from build123d import *

# Parameters (mm, degrees)
ESQUISSE1_R                                = 30
BOSS_EXTRU_1_DEPTH                         = 15
ESQUISSE2_R                                = 12.5
BOSS_EXTRU_2_DEPTH                         = 69
ESQUISSE4_2_W                              = 230
ESQUISSE4_2_H                              = 40
ENL_V_MAT_EXTRU_1_DEPTH                    = 5
CHAMBRAGE_POUR_VIS_T_TE_HEXAGONALE_2_COUNT = 2
CHAMBRAGE_POUR_VIS_T_TE_HEXAGONALE_2_PITCH = 41
ESQUISSE17_R                               = 6
BOSS_EXTRU_4_DEPTH                         = 88.38
ESQUISSE18_W                               = 10.356322474
ESQUISSE18_H                               = 3
ENL_V_MAT_EXTRU_2_DEPTH                    = 3


with BuildPart() as part:
    # Esquisse1 → Boss.-Extru.1 (new body)
    with BuildSketch(Plane.XY):
        Circle(ESQUISSE1_R)
    extrude(amount=BOSS_EXTRU_1_DEPTH)

    # Esquisse2 → Boss.-Extru.2 (add)
    with BuildSketch(Plane(origin=(0, 0, 0), x_dir=(-1, 0, 0), z_dir=(0, 0, -1))):
        with Locations(Location((0, 0, 0), (0, 0, 180))):
            Circle(ESQUISSE2_R)
    extrude(amount=BOSS_EXTRU_2_DEPTH)

    # Esquisse4<2> → Enlèv. mat.-Extru.1 (cut)
    with BuildSketch(Plane.XY.offset(15)):
        Rectangle(ESQUISSE4_2_W, ESQUISSE4_2_H)
    extrude(amount=-ENL_V_MAT_EXTRU_1_DEPTH, mode=Mode.SUBTRACT)

    # Esquisse14 → Chambrage pour vis à tête hexagonale M51 (revolve, cut)
    with BuildSketch(Plane.YZ.offset(-20.5)):
        Polygon((0, 0), (0, 15), (2.75, 15), (2.75, 3.605), (2.775, 3.58), (6.12, 3.58), (6.12, 0), align=None)
    chambrage_pour_vis_t_te_hexagonale_m51 = revolve(axis=Axis((-20.5, 0, -6.35), (0, 0, 1)), mode=Mode.SUBTRACT)

    # Chambrage pour vis _ t_te hexagonale 2: Chambrage pour vis à tête hexagonale M51 ×2
    with Locations(*[(i * CHAMBRAGE_POUR_VIS_T_TE_HEXAGONALE_2_PITCH, 0, 0) for i in range(1, CHAMBRAGE_POUR_VIS_T_TE_HEXAGONALE_2_COUNT)]):
        add(chambrage_pour_vis_t_te_hexagonale_m51, mode=Mode.SUBTRACT)

    # Esquisse17 → Boss.-Extru.4 (add)
    with BuildSketch(Plane(origin=(0, 0, -69), x_dir=(-1, 0, 0), z_dir=(0, 0, -1))):
        Circle(ESQUISSE17_R)
    extrude(amount=BOSS_EXTRU_4_DEPTH)

    # Esquisse18 → Enlèv. mat.-Extru.2 (cut)
    with BuildSketch(Plane(origin=(0, 0, -157.38), x_dir=(-1, 0, 0), z_dir=(0, 0, -1))):
        with Locations((1.787207702, 0)):
            Rectangle(ESQUISSE18_W, ESQUISSE18_H)
    extrude(amount=-ENL_V_MAT_EXTRU_2_DEPTH, mode=Mode.SUBTRACT)


solid = part.part
Design review of the part built by this model. Coordinates are the model's own, in mm. A direction names the side the tool comes from. Coordinates: 2 decimals unless noted, no trailing zeros. Loops run counter-clockwise (first coordinate to the right, second up) from the corner with the lowest first, then second, coordinate; pieces in that order, holes last. Notation, with made-up numbers: (-32.5, 78) -> (-23.5, 78) arc R18 ccw to (-23.5, 89) -> close; hole circle Ø10 at (3, 84). An arc over 180 degrees is marked (long way). Use a Markdown table: item, result. Add a question column.
Item 1: We need section D-D, the plane y = -15.5. Write out the cut boundary in (x, z), and give its area (3 significant figures).
Item 2: Clearance check with flat-ended pins moving along their axes: P1, Ø3.5, axis at y = 0.5, z = -155.5, coming from the -X side; P2, Ø13.5, axis at x = 23.5, y = 2.5, coming from the -Z side; P3, Ø2, axis at x = -4.5, z = -49, coming from the -Y side; P4, Ø5, axis at x = -2, y = 0.5, coming from the -Z side. State where each tip first meets the part, or that it passes through.
Item 3: Wall thickness on L1, parallel to X at y = 0, z = 1.3; L2, parallel to X at y = 0, z = 6.5; L3, parallel to Y at x = -20, z = 2: over which ranges is each line inside the solid? List them lowest first. Write a range as from..to.
Item 4: We need section B-B, the plane x = 0. Write out the cut boundary in (y, z).
Item 5: The part is to be moulded in two halves that separate along Y. For faces 4 (the cylindrical face through (11.923, -3.755, -34.017)), 5 (the flat face through (0, -13, 0)), 6 (the flat face through (-1, 0, -154.38)), 7 (the cylindrical face through (-14.526, -1.327, 1.765)), say which applies: +Y half, -Y half, draft (parallel to the pull), parting line (faces both ways), or undercut.
Item 6: Machinability: for faces 1 (the flat face through (-3, 5.4, -69)), 2 (the flat face through (0, 0, 10)), 3 (the flat face through (3.391, 0, -156)), which of the approach directions +Z, -Z, +X, -X, +Y, -Y give a long, thin tool a straight path to every point of the face, cutting with its end or side? Answer none if there is none.
Item 7: We need section A-A, the plane x = -20.5. Write out the cut boundary in (y, z) (3 decimals), and give its area (3 significant figures).
Item 8: We need section C-C, the plane z = -119.5. Write out the cut boundary in (x, y).
Numbers:
| question | item | result |
|---|---|---|
| 1 | outline | (-25.69, 0) -> (25.69, 0) -> (25.69, 10) -> (-25.69, 10) -> close |
| 1 | area | 514 mm^2 |
| 2 | P1 | stops at x = -6 |
| 2 | P2 | stops at z = 0 |
| 2 | P3 | stops at y = -12 |
| 2 | P4 | stops at z = -157.38 |
| 3 | L1 | x = -30..-26.62, -14.38..14.38, 26.62..30 |
| 3 | L2 | x = -30..-23.25, -17.75..17.75, 23.25..30 |
| 3 | L3 | y = -22.36..-6.1, 6.1..22.36 |
| 4 | outline | (-30, 0) -> (-12.5, 0) -> (-12.5, -69) -> (-6, -69) -> (-6, -157.38) -> (-1.5, -157.38) -> (-1.5, -154.38) -> (1.5, -154.38) -> (1.5, -157.38) -> (6, -157.38) -> (6, -69) -> (12.5, -69) -> (12.5, 0) -> (30, 0) -> (30, 15) -> (20, 15) -> (20, 10) -> (-20, 10) -> (-20, 15) -> (-30, 15) -> close |
| 5 | face 4 | parting line |
| 5 | face 5 | draft |
| 5 | face 6 | undercut |
| 5 | face 7 | undercut |
| 6 | face 1 | -Z |
| 6 | face 2 | +Z, +X, -X |
| 6 | face 3 | -Z, -X |
| 7 | outline | (-21.903, 0) -> (-6.12, 0) -> (-6.12, 3.58) -> (-2.775, 3.58) -> (-2.75, 3.605) -> (-2.75, 10) -> (-20, 10) -> (-20, 15) -> (-21.903, 15) -> close; (2.75, 3.605) -> (2.775, 3.58) -> (6.12, 3.58) -> (6.12, 0) -> (21.903, 0) -> (21.903, 15) -> (20, 15) -> (20, 10) -> (2.75, 10) -> close |
| 7 | area | 378 mm^2 |
| 8 | outline | circle Ø12 at (0, 0) |
